```python
from build123d import *

# Parameters (mm, degrees)
F0_W     = 53.126359
F0_H     = 31.090025
F1_DEPTH = 25
F2_SIZE  = 5
F3_T     = -5
F5_D     = 12


with BuildPart() as f1:
    # F0 (on Front) → F1 (new body)
    with BuildSketch(Plane.XZ):
        with Locations((-32.712854, -4.270607)):
            Rectangle(F0_W, F0_H)
    extrude(amount=F1_DEPTH)

    # F2
    f2_edges = [f1.edges().sort_by_distance(p)[0] for p in [
        (-6.149674, -12.5, 11.274405),
        (-59.276033, -12.5, 11.274405),
        (-6.149674, -12.5, -19.81562),
        (-59.276033, -12.5, -19.81562),
    ]]
    chamfer(f2_edges, length=F2_SIZE)

    # F3
    f3_openings = [f1.faces().sort_by_distance(p)[0] for p in [
        (-32.712854, -25, -4.270608),
    ]]
    offset(amount=F3_T, openings=f3_openings)

    # F5 (through all)
    with Locations(Plane.XY.offset(11.274405)):
        with Locations((-37.922993, -10.591106)):
            Hole(F5_D / 2)


solid = f1.part
```
Work out the finished part from the listing and answer in its coordinate system (mm). A direction names the side the tool comes from. Give positions to 0.01 mm unless a question says otherwise; leave off trailing zeros. Order: outer loops, then holes, each group sorted by start corner. A loop starts at its lowest first (then second) coordinate and runs counter-clockwise, first axis right, second up. Notation, with made-up numbers: (49, 36) - (93, 36) arc R17 ccw to (93, 69) - close; hole circle Ø8 at (-38.5, 42.5). An arc over 180 degrees is marked (long way). One line per item, written item: value. Start each with the question number.
1. Each of these flat-tipped pins is pushed along its axis until it touches: pin 1 Ø7 at (x, z) = (-47.5, -2.5) entering from -Y; pin 2 Ø9.5 at (x, y) = (-37.92, -10.59) entering from -Z. Where does it stop, or does it pass through?
2. Section C-C, the plane x = -33.5 is taken. Write down the section's boundary in (y, z), then the cut area to 3 significant figures.
3. Section A-A, the plane y = -21.75 is taken. Write down the section's boundary in (x, z).
4. Section D-D, the plane y = -3.25 is taken. Write down the section's boundary in (x, z).
5. Section B-B, the plane z = 2 is taken. Write down the section's boundary in (x, y).
6. Which of the six approach directions +Z, -Z, +X, -X, +Y, -Y give full straight-line access (tool end or side, diameter ignored) to faces 4 (the face through (-56.74, -12.32, -17.35)), 5 (the face through (-53.23, -14.86, 5.25))?
7. Consider line 1 (Z direction, x = -50.5, y = -22.25); line 2 (X direction, y = -18.5, z = -5); line 3 (Y direction, x = -18, z = -1). Determine where each line is inside the solid, lowest interval first.
8. For a pull along Y with two mould halves and no side action, classify faces 1 (the face through (-33, -15, 11.274)), 2 (the face through (-24, -5, -4)), 3 (the face through (-37.142, -4.642, -7.943)) as released by +Y, released by -Y, zero draft, split by the parting line, or undercut.
Filled sheet:
1. pin 1: y = -5
1. pin 2: through
2. outline: (-25, -19.82) - (-14.65, -19.82) - (-14.65, -14.82) - (-25, -14.82) - close; (-25, 6.27) - (-14.65, 6.27) - (-14.65, 11.27) - (-25, 11.27) - close; (-6.54, -19.82) - (0, -19.82) - (0, 11.27) - (-6.54, 11.27) - (-6.54, 6.27) - (-5, 6.27) - (-5, -14.82) - (-6.54, -14.82) - close
2. area: 274 mm²
3. outline: (-59.28, -14.82) - (-54.28, -19.82) - (-11.15, -19.82) - (-6.15, -14.82) - (-6.15, 6.27) - (-11.15, 11.27) - (-54.28, 11.27) - (-59.28, 6.27) - close; hole (-54.28, -12.74) - (-52.2, -14.82) - (-13.22, -14.82) - (-11.15, -12.74) - (-11.15, 4.2) - (-13.22, 6.27) - (-52.2, 6.27) - (-54.28, 4.2) - close
4. outline: (-59.28, -14.82) - (-54.28, -19.82) - (-11.15, -19.82) - (-6.15, -14.82) - (-6.15, 6.27) - (-11.15, 11.27) - (-54.28, 11.27) - (-59.28, 6.27) - close
5. outline: (-59.28, -25) - (-54.28, -25) - (-54.28, -5) - (-40.1, -5) arc R6 cw to (-35.75, -5) - (-11.15, -5) - (-11.15, -25) - (-6.15, -25) - (-6.15, 0) - (-59.28, 0) - close
6. face 4: -Z, -X, +Y, -Y
6. face 5: -Y
7. line 1: -19.82 to -14.82, 6.27 to 11.27
7. line 2: -59.28 to -54.28, -11.15 to -6.15
7. line 3: -5 to 0
8. face 1: zero draft
8. face 2: released by -Y
8. face 3: undercut
